Check sheet for the modelled part. Datum: model origin and axes. Units: mm. A direction names the side the tool comes from. Round coordinates to 2 decimals unless told otherwise and drop trailing zeros. Answer in a Markdown table with one row per item.
from build123d import *

# Parameters (mm, degrees)
F1_DEPTH = 14.478
F5_R     = 23.6640826147
F6_DEPTH = 1.1938
F5_R_2   = 5.4611807343
F7_DEPTH = 18.034
F8_DEPTH = 3.3782
F9_R     = 1.016


with BuildPart() as f1:
    # F0 (on Top) → F1 (new body)
    with BuildSketch(Plane.XY):
        with BuildLine():
            Line((-30.3200407773, 22.6429850771), (-24.6294784274, 13.5667208411))
            ThreePointArc((-24.6294784274, 13.5667208411), (-25.9783872248, 10.7606003171), (-27.0087915183, 7.8225509079))
            Line((-27.0087915183, 7.8225509079), (-37.4505147338, 5.4284981452))
            Line((-37.4505147338, 5.4284981452), (-37.4505147338, -5.4284981452))
            Line((-37.4505147338, -5.4284981452), (-27.0087915183, -7.8225509079))
            ThreePointArc((-27.0087915183, -7.8225509079), (-25.9783872248, -10.7606003171), (-24.6294784274, -13.5667208411))
            Line((-24.6294784274, -13.5667208411), (-30.3200407773, -22.6429850771))
            Line((-30.3200407773, -22.6429850771), (-22.6429850771, -30.3200407773))
            Line((-22.6429850771, -30.3200407773), (-13.5667208411, -24.6294784274))
            ThreePointArc((-13.5667208411, -24.6294784274), (-10.7606003171, -25.9783872248), (-7.8225509079, -27.0087915183))
            Line((-7.8225509079, -27.0087915183), (-5.4284981452, -37.4505147338))
            Line((-5.4284981452, -37.4505147338), (5.4284981452, -37.4505147338))
            Line((5.4284981452, -37.4505147338), (7.8225509079, -27.0087915183))
            ThreePointArc((7.8225509079, -27.0087915183), (10.7606003171, -25.9783872248), (13.5667208411, -24.6294784274))
            Line((13.5667208411, -24.6294784274), (22.6429850771, -30.3200407773))
            Line((22.6429850771, -30.3200407773), (30.3200407773, -22.6429850771))
            Line((30.3200407773, -22.6429850771), (24.6294784274, -13.5667208411))
            ThreePointArc((24.6294784274, -13.5667208411), (25.9783872248, -10.7606003171), (27.0087915183, -7.8225509079))
            Line((27.0087915183, -7.8225509079), (37.4505147338, -5.4284981452))
            Line((37.4505147338, -5.4284981452), (37.4505147338, 5.4284981452))
            Line((37.4505147338, 5.4284981452), (27.0087915183, 7.8225509079))
            ThreePointArc((27.0087915183, 7.8225509079), (25.9783872248, 10.7606003171), (24.6294784274, 13.5667208411))
            Line((24.6294784274, 13.5667208411), (30.3200407773, 22.6429850771))
            Line((30.3200407773, 22.6429850771), (22.6429850771, 30.3200407773))
            Line((22.6429850771, 30.3200407773), (13.5667208411, 24.6294784274))
            ThreePointArc((13.5667208411, 24.6294784274), (10.7606003171, 25.9783872248), (7.8225509079, 27.0087915183))
            Line((7.8225509079, 27.0087915183), (5.4284981452, 37.4505147338))
            Line((5.4284981452, 37.4505147338), (-5.4284981452, 37.4505147338))
            Line((-5.4284981452, 37.4505147338), (-7.8225509079, 27.0087915183))
            ThreePointArc((-7.8225509079, 27.0087915183), (-10.7606003171, 25.9783872248), (-13.5667208411, 24.6294784274))
            Line((-13.5667208411, 24.6294784274), (-22.6429850771, 30.3200407773))
            Line((-22.6429850771, 30.3200407773), (-30.3200407773, 22.6429850771))
        make_face()
    extrude(amount=F1_DEPTH)

    # F3 (on Front) → F4 (revolve, cut)
    with BuildSketch(Plane.XZ):
        Polygon((-39.187733084, 17.5162125379), (-39.187733084, 9.2955380678), (-23.6767126761, 14.478), (-23.6767126761, 17.5162125379), align=None)
    revolve(axis=Axis((0, 0, 21.3634204119), (0, 0, 1)), mode=Mode.SUBTRACT)

    # F5 (on face) → F6 (cut)
    with BuildSketch(Plane.XY.offset(14.478)):
        Circle(F5_R)
        with BuildLine():
            ThreePointArc((-19.6771575376, 0), (-13.9138515293, 13.9138515293), (0, 19.6771575376))
            Line((0, 19.6771575376), (0, 17.0739562129))
            ThreePointArc((0, 17.0739562129), (12.0731102199, 12.0731102199), (17.0739562129, 0))
            Line((17.0739562129, 0), (19.6771575376, 0))
            ThreePointArc((19.6771575376, 0), (13.9138515293, -13.9138515293), (0, -19.6771575376))
            Line((0, -19.6771575376), (0, -17.0739562129))
            ThreePointArc((0, -17.0739562129), (-12.0731102199, -12.0731102199), (-17.0739562129, 0))
            Line((-17.0739562129, 0), (-19.6771575376, 0))
        make_face(mode=Mode.SUBTRACT)
    extrude(amount=-F6_DEPTH, mode=Mode.SUBTRACT)

    # F5 (on face) → F7 (cut)
    with BuildSketch(Plane.XY.offset(14.478)):
        Circle(F5_R_2)
    extrude(amount=-F7_DEPTH, mode=Mode.SUBTRACT)

    # F5 (on face) → F8 (cut)
    with BuildSketch(Plane.XY.offset(14.478)):
        with BuildLine():
            Line((0, 8.8564318695), (0, 14.0838984666))
            ThreePointArc((0, 14.0838984666), (-9.9588201113, -9.9588201113), (14.0838984666, 0))
            Line((14.0838984666, 0), (8.8564318695, 0))
            ThreePointArc((8.8564318695, 0), (-6.262443032, -6.262443032), (0, 8.8564318695))
        make_face()
    extrude(amount=-F8_DEPTH, mode=Mode.SUBTRACT)

    # F9
    f9_edges = [f1.edges().sort_by_distance(p)[0] for p in [
        (-37.450515, -5.428498, 4.8726),
        (-37.450515, 5.428498, 4.8726),
        (-30.320041, -22.642985, 4.8726),
        (-22.642985, -30.320041, 4.8726),
        (-5.428498, -37.450515, 4.8726),
        (5.428498, -37.450515, 4.8726),
        (22.642985, -30.320041, 4.8726),
        (30.320041, -22.642985, 4.8726),
        (37.450515, -5.428498, 4.8726),
        (37.450515, 5.428498, 4.8726),
        (30.320041, 22.642985, 4.8726),
        (22.642985, 30.320041, 4.8726),
        (5.428498, 37.450515, 4.8726),
        (-5.428498, 37.450515, 4.8726),
        (-30.320041, 22.642985, 4.8726),
        (-22.642985, 30.320041, 4.8726),
        (19.677158, 0, 13.8811),
        (17.073956, 0, 13.8811),
        (0, 17.073956, 13.8811),
        (0, 19.677158, 13.8811),
        (-5.461181, 0, 14.478),
        (-19.677158, 0, 13.8811),
        (-17.073956, 0, 13.8811),
        (0, -19.677158, 13.8811),
        (0, -17.073956, 13.8811),
    ]]
    fillet(f9_edges, radius=F9_R)


solid = f1.part
Item 1: Set-up check for faces 4 (the flat face through (27.22, 17.7, 6.41)), 5 (the cylindrical face through (-10.72, 25.995, 6.406)), 6 (the cylindrical face through (-25.96, 10.8, 6.41)), 7 (the cylindrical face through (14.056, -13.771, 13.889)): record each of +Z, -Z, +X, -X, +Y, -Y from which the full face is reachable in a straight line by a thin tool's end or side.
Result sheet:
| item | result |
|---|---|
| face 4 | +Z, -Z, +X |
| face 5 | +Z, -Z, +Y |
| face 6 | +Z, -Z, -X |
| face 7 | +Z |
Item 2: Scan lines: line 1 (Y direction, x = -28.5, z = 7.5); line 2 (X direction, y = 29.5, z = 3.75); line 3 (Y direction, x = -25.5, z = 6). Record each from-to range of solid material in increasing order. Write a range as [from, to].
Result sheet:
| item | result |
|---|---|
| line 1 | y = [-24.46, -19.74], [-7.48, 7.48], [19.74, 24.46] |
| line 2 | x = [-23.46, -21.34], [-7.25, 7.25], [21.34, 23.46] |
| line 3 | y = [-27.46, -14.96], [-11.85, 11.85], [14.96, 27.46] |
Item 3: Depth check by flat-ended pin: P1, Ø6.5, axis at x = 0, y = 0, coming from the +Z side; P2, Ø3.5, axis at y = 12, z = 13.5, coming from the -X side; P3, Ø6, axis at x = 14.5, z = 1.5, coming from the +Y side; P4, Ø1.7, axis at x = 12, z = 12, coming from the -Y side. Enter the tip coordinate at first touch or a pass-through.
Result sheet:
| item | result |
|---|---|
| P1 | passes through |
| P2 | stops at x = -26.15 |
| P3 | stops at y = 27.1 |
| P4 | stops at y = -25.81 |
Item 4: Cross-section at A-A (x = -28). State how many separate pieces and enclosed holes the cut face has, and give its area (3 significant figures).
Result sheet:
| item | result |
|---|---|
| separate pieces | 3 |
| enclosed holes | 0 |
| area | 323 mm^2 |
Item 5: Mould release check, pull along Y, two halves, no side actions. Record for faces 1 (the cylindrical face through (-5.13, -23.1, 13.89)), 2 (the flat face through (-26.527, -26.436, 4.869)), 3 (the flat face through (17.821, 27.297, 6.406)): pulls with the +Y half, pulls with the -Y half, needs draft (parallel to the pull), parting line crosses it, or undercut.
Result sheet:
| item | result |
|---|---|
| face 1 | undercut |
| face 2 | pulls with the -Y half |
| face 3 | pulls with the +Y half |
